Part model, mm, in its own coordinate system. A direction names the side the tool comes from. Give positions to 0.01 mm unless a question says otherwise; leave off trailing zeros. Loops run counter-clockwise (first coordinate to the right, second up) from the corner with the lowest first, then second, coordinate; pieces in that order, holes last. Notation, with made-up numbers: (50, 69) -> (71, 69) arc R32 cw to (71, 107) -> close; hole circle Ø1 at (2, 30.5). An arc over 180 degrees is marked (long way). Write item = value, one per line.
from build123d import *

# Parameters (mm, degrees)
SKETCH1_W                    = 40
SKETCH1_H                    = 80
BOSS_EXTRUDE1_DEPTH          = 59
SKETCH2_R                    = 11
SKETCH2_R_2                  = 2.5
CUT_EXTRUDE1_DEPTH           = 77.829612465
SKETCH5_R                    = 2.55
CUT_EXTRUDE3_DEPTH           = 5
FILLET3_R                    = 10
FILLET4_R                    = 10
F_7_0_7_DIAMETER_HOLE1_D     = 7
F_7_0_7_DIAMETER_HOLE1_DEPTH = 4.896987833
F_7_0_7_DIAMETER_HOLE1_TIP   = 2.103012167
SKETCH13_W                   = 10
SKETCH13_H                   = 48.48
BOSS_EXTRUDE2_DEPTH          = 50
SKETCH18_W                   = 6.2
SKETCH18_H                   = 6.9
CUT_EXTRUDE4_DEPTH           = 103.023881602
F_5_0_5_DIAMETER_HOLE1_D     = 5
F_5_0_5_DIAMETER_HOLE1_DEPTH = 18.497848452
F_5_0_5_DIAMETER_HOLE1_TIP   = 1.502151548


with BuildPart() as part:
    # Sketch1 → Boss-Extrude1 (new body)
    with BuildSketch(Plane.XY):
        with Locations((0.060830656, -4.937205352)):
            Rectangle(SKETCH1_W, SKETCH1_H)
    extrude(amount=BOSS_EXTRUDE1_DEPTH)

    # Sketch2 → Cut-Extrude1 (cut, through all)
    with BuildSketch(Plane.XY):
        Circle(SKETCH2_R)
        with Locations((-11.313708499, 11.313708499)):
            Circle(SKETCH2_R_2)
        with Locations((-0.122338904, 15.759725587)):
            Circle(SKETCH2_R_2)
        with Locations((11.402693442, 11.263696484)):
            Circle(SKETCH2_R_2)
        with Locations((11.339369089, -11.406422087)):
            Circle(SKETCH2_R_2)
        with Locations((-0.312311964, -16.029099896)):
            Circle(SKETCH2_R_2)
        with Locations((-11.204100775, -11.406422087)):
            Circle(SKETCH2_R_2)
    extrude(amount=CUT_EXTRUDE1_DEPTH, mode=Mode.SUBTRACT)

    # Sketch5 → Cut-Extrude3 (cut)
    with BuildSketch(Plane.ZY.offset(19.939169344)):
        with Locations((29.5, -4.937205352)):
            Circle(SKETCH5_R)
        with Locations((39.5, -4.937205352)):
            Circle(SKETCH5_R)
        with Locations((19.5, -4.937205352)):
            Circle(SKETCH5_R)
        with Locations((29.5, 5.062794648)):
            Circle(SKETCH5_R)
        with Locations((29.5, -14.937205352)):
            Circle(SKETCH5_R)
    extrude(amount=-CUT_EXTRUDE3_DEPTH, mode=Mode.SUBTRACT)

    # Fillet3
    fillet3_edges = [part.edges().sort_by_distance(p)[0] for p in [
        (-19.939169344, -44.937205352, 29.5),
    ]]
    fillet(fillet3_edges, radius=FILLET3_R)

    # Fillet4
    fillet4_edges = [part.edges().sort_by_distance(p)[0] for p in [
        (-19.939169344, 35.062794648, 29.5),
    ]]
    fillet(fillet4_edges, radius=FILLET4_R)

    # Ø7.0 (7) Diameter Hole1
    with Locations(Plane(origin=(20.060830656, 0, 0), x_dir=(0, 0, -1), z_dir=(1, 0, 0))):
        with Locations((-52.5, -26.937205352), (-52.5, -39.937205352), (-6.5, -39.937205352), (-6.5, -26.937205352)):
            Hole(F_7_0_7_DIAMETER_HOLE1_D / 2, depth=F_7_0_7_DIAMETER_HOLE1_DEPTH)
            with Locations((0, 0, -(F_7_0_7_DIAMETER_HOLE1_DEPTH + F_7_0_7_DIAMETER_HOLE1_TIP / 2))):  # 118° drill point
                Cone(0, F_7_0_7_DIAMETER_HOLE1_D / 2, F_7_0_7_DIAMETER_HOLE1_TIP, mode=Mode.SUBTRACT)

    # Sketch13 → Boss-Extrude2 (add)
    with BuildSketch(Plane(origin=(20.060830656, 0, 0), x_dir=(0, 0, -1), z_dir=(1, 0, 0))):
        with Locations((-5, 3.922794648)):
            Rectangle(SKETCH13_W, SKETCH13_H)
        with Locations((-54, 3.922794648)):
            Rectangle(SKETCH13_W, SKETCH13_H)
    extrude(amount=BOSS_EXTRUDE2_DEPTH)

    # Sketch18 → Cut-Extrude4 (cut, through all)
    with BuildSketch(Plane(origin=(0, 0, 0), x_dir=(-1, 0, 0), z_dir=(0, 0, -1))):
        with Locations((-16.960830656, 31.612794648)):
            Rectangle(SKETCH18_W, SKETCH18_H)
    extrude(amount=-CUT_EXTRUDE4_DEPTH, mode=Mode.SUBTRACT)

    # Ø5.0 (5) Diameter Hole1
    with Locations(Plane(origin=(0, 28.162794648, 0), x_dir=(1, 0, 0), z_dir=(0, 1, 0))):
        with Locations((18.490830656, -5.94), (65.630830656, -5.94), (65.630830656, -53.06), (18.490830656, -53.06)):
            Hole(F_5_0_5_DIAMETER_HOLE1_D / 2, depth=F_5_0_5_DIAMETER_HOLE1_DEPTH)
            with Locations((0, 0, -(F_5_0_5_DIAMETER_HOLE1_DEPTH + F_5_0_5_DIAMETER_HOLE1_TIP / 2))):  # 118° drill point
                Cone(0, F_5_0_5_DIAMETER_HOLE1_D / 2, F_5_0_5_DIAMETER_HOLE1_TIP, mode=Mode.SUBTRACT)


solid = part.part
1) Drill centre lines: line 1 along X through (y, z) = (19, 53); line 2 along Y through (x, z) = (-17, 29); line 3 along Y through (x, z) = (-1, 23). Where is each one in solid material? Low to high. Write a range as [from, to].
Resolved:
line_1 = [-19.94, 15.99], [20.99, 63.13], [68.13, 70.06]
line_2 = [-42.02, -17.44], [-12.44, -7.44], [-2.44, 2.56], [7.56, 32.14]
line_3 = [-44.94, -18.43], [-13.63, -10.95], [10.95, 13.42], [18.1, 35.06]
2) Slice it at D-D, the plane x = 0. List the corners of the cut face in (y, z).
Resolved:
outline = (-44.94, 0) -> (-18.51, 0) -> (-18.51, 59) -> (-44.94, 59) -> close; (-13.55, 0) -> (-11, 0) -> (-11, 59) -> (-13.55, 59) -> close; (11, 0) -> (13.26, 0) -> (13.26, 59) -> (11, 59) -> close; (18.26, 0) -> (35.06, 0) -> (35.06, 59) -> (18.26, 59) -> close
3) Slice it at C-C, the plane z = 40. List the corners of the cut face in (x, y), and give its area (3 significant figures).
Resolved:
outline = (-19.94, -34.94) arc R10 ccw to (-9.94, -44.94) -> (20.06, -44.94) -> (20.06, 28.16) -> (13.86, 28.16) -> (13.86, 35.06) -> (-9.94, 35.06) arc R10 ccw to (-19.94, 25.06) -> (-19.94, -2.44) -> (-14.94, -2.44) -> (-14.94, -7.44) -> (-19.94, -7.44) -> close; hole circle Ø5 at (-11.31, 11.31); hole circle Ø5 at (-11.2, -11.41); hole circle Ø22 at (0, 0); hole circle Ø5 at (-0.31, -16.03); hole circle Ø5 at (-0.12, 15.76); hole circle Ø5 at (11.34, -11.41); hole circle Ø5 at (11.4, 11.26)
area = 2,590 mm²
4) Slice it at B-B, the plane x = 27.5. List the corners of the cut face in (y, z), and give its area (3 significant figures).
Resolved:
outline = (-20.32, 0) -> (28.16, 0) -> (28.16, 10) -> (-20.32, 10) -> close; (-20.32, 49) -> (28.16, 49) -> (28.16, 59) -> (-20.32, 59) -> close
area = 970 mm²
5) Which spindle directions (+Z, -Z, +X, -X, +Y, -Y) get a long thin tool onto all of the face, cutting with end or side? Do faces 3 (the face through (17.578, -36.467, 6.044)), 4 (the face through (45, 4, 49)), 5 (the face through (-17.09, -41.93, 29.91)), 6 (the face through (-14.939, -5, 39)). Say none if no direction does.
Resolved:
face_3 = +X
face_4 = +X, +Y, -Y
face_5 = +Z, -Z, -X, -Y
face_6 = -X
6) Slice it at A-A, the plane y = 0. List the corners of the cut face in (x, z), and give its area (3 significant figures).
Resolved:
outline = (-19.94, 0) -> (-11, 0) -> (-11, 59) -> (-19.94, 59) -> close; (11, 0) -> (70.06, 0) -> (70.06, 10) -> (20.06, 10) -> (20.06, 49) -> (70.06, 49) -> (70.06, 59) -> (11, 59) -> close
area = 2,060 mm²
7) Drop flat-ended pins along their axis: P1, Ø4, axis at y = -39.94, z = 6.5, coming from the +X side; P2, Ø2, axis at y = 12, z = 44, coming from the +X side; P3, Ø10, axis at x = 23.5, z = 33.5, coming from the +Y side. Give the stop position or say it passes through.
Resolved:
P1 = 14.26
P2 = 20.06
P3 = 28.16
8) Pull direction Z, two halves, no side cores. Call faces 1 (the face through (17.578, -23.467, 6.044)), 2 (the face through (-10.051, -13.624, 29.087)): pulls with the +Z half, pulls with the -Z half, needs draft (parallel to the pull), parting line crosses it, or undercut.
Resolved:
face_1 = undercut
face_2 = needs draft
